```python
from build123d import *

# Parameters (mm, degrees)
CUT_EXTRUDE1_DEPTH = 1.5
FILLET1_R          = 0.5


with BuildPart() as part:
    # Sketch1 → Revolve1 (revolve)
    with BuildSketch(Plane.XY, mode=Mode.PRIVATE) as revolve1_sk:
        Polygon((15.7, 0), (15.7, 1.4), (1.7, 1.4), (1.7, 2.75), (1, 2.75), (0, 1.5), (0, 0), align=None)
    revolve(revolve1_sk.sketch.rotate(Axis((0, 0, 0), (1, 0, 0)), 180), axis=Axis((0, 0, 0), (1, 0, 0)))

    # Sketch2 → Cut-Extrude1 (cut)
    with BuildSketch(Plane.ZY):
        Polygon((1.154700538, 0), (0.577350269, 1), (-0.577350269, 1), (-1.154700538, 0), (-0.577350269, -1), (0.577350269, -1), align=None)
    extrude(amount=-CUT_EXTRUDE1_DEPTH, mode=Mode.SUBTRACT)

    # Fillet1
    fillet1_edges = [part.edges().sort_by_distance(p)[0] for p in [
        (1, 2.75, 0),
        (0, 1.5, 0),
    ]]
    fillet(fillet1_edges, radius=FILLET1_R)


solid = part.part
```
Verification items for the finished model (mm, model axes). A direction names the side the tool comes from. Give positions to 0.01 mm unless a question says otherwise; leave off trailing zeros. Order: outer loops, then holes, each group sorted by start corner. A loop starts at its lowest first (then second) coordinate and runs counter-clockwise, first axis right, second up. Notation, with made-up numbers: M 11,71 L 42,71 A22 ccw 42,84 Z; hole C 87,10.25 d11. An arc over 180 degrees is marked long. Answer in a Markdown table with one row per item. Add a question column.
Item 1: Scan lines: probe 1 along Y at (x, z) = (6.5, -0.1); probe 2 along X at (y, z) = (-0.5, 0.4); probe 3 along Y at (x, z) = (1.25, -1). Record each from-to range of solid material in increasing order. Write a range as from..to.
Item 2: Gauge pin test, flat ends, axial feed: pin 1 (1.5 mm diameter, centred on x = 8, z = -0.5, fed in from -Y); pin 2 (0.6 mm diameter, centred on x = 0.5, z = 0, fed in from -Y). Record the tip position at first contact, or that the pin passes through.
Item 3: Mould release check, pull along Z, two halves, no side actions. Record for faces 3 (the flat face through (1, -1, 0)), 4 (the flat face through (15.7, 0, 0)), 5 (the cylindrical face through (1.467, 0.596, 2.685)), 6 (the flat face through (0.74, -0.51, 0.86)): released by +Z, released by -Z, zero draft, split by the parting line, or undercut.
Item 4: Section check A-A, the plane x = 14.5. Enter the section's corners in (y, z), and give its area (3 significant figures).
Item 5: Tool access check on faces 1 (the flat face through (1.7, 1.2, 1.2)), 2 (the flat face through (1.5, 0, 0)). Record the directions out of +Z, -Z, +X, -X, +Y, -Y that give a thin tool (end or side, any length) a straight path to the whole face; none if there is none.
Filled sheet:
| question | item | result |
|---|---|---|
| 1 | probe 1 | y = -1.4..1.4 |
| 1 | probe 2 | x = 1.5..15.7 |
| 1 | probe 3 | y = -2.56..-0.27, 0.27..2.56 |
| 2 | pin 1 | stops at y = -1.4 |
| 2 | pin 2 | stops at y = -2.5 |
| 3 | face 3 | undercut |
| 3 | face 4 | zero draft |
| 3 | face 5 | split by the parting line |
| 3 | face 6 | undercut |
| 4 | outline | C 0,0 d2.8 |
| 4 | area | 6.16 mm^2 |
| 5 | face 1 | +X |
| 5 | face 2 | -X |
